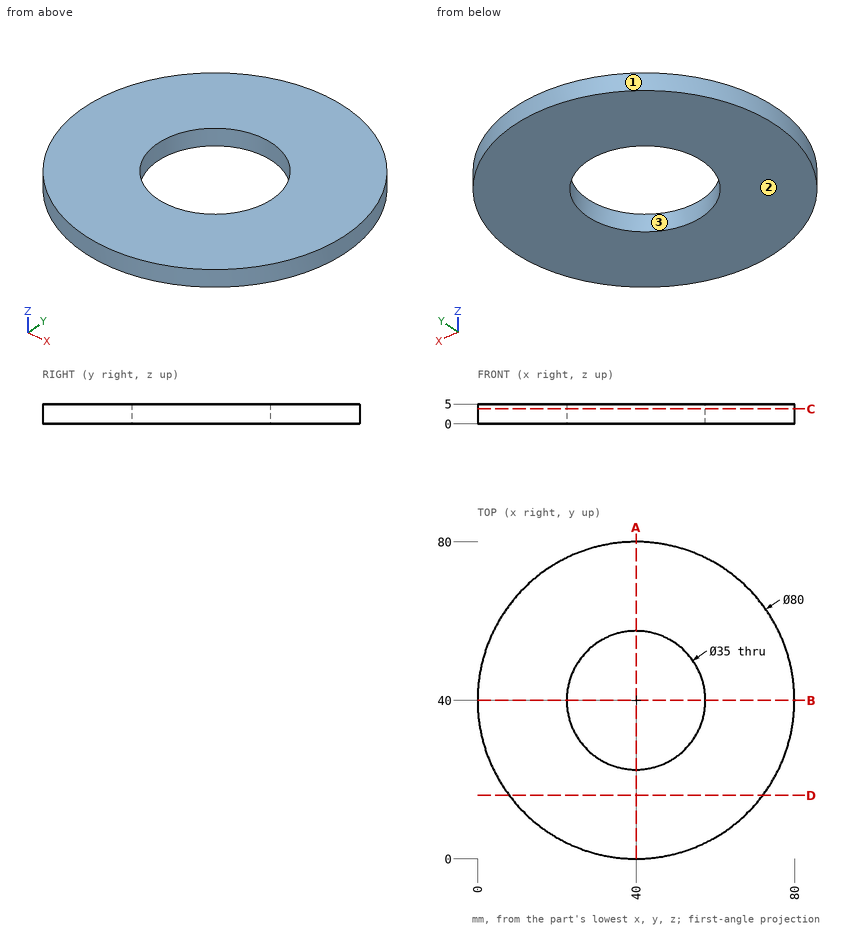
Print and shaded views of the part. All mm, measured from the part's lowest x, y and z. Round coordinates to 2 decimals unless told otherwise and drop trailing zeros. Write each loop counter-clockwise with the first axis right and the second up, starting at its lowest first coordinate (ties: lowest second). Pieces come first, ordered by that corner, then holes. Notation, with made-up numbers: (52.5, 32.25) - (81.5, 32.25) arc R22 ccw to (81.5, 52.25) - close; hole circle Ø7 at (7, -32). An arc over 180 degrees is marked (long way). Write each question's results on one line, items separated by ' | '. Start each with the question number.
Item 1: Drop flat-ended pins along their axis: P1, Ø1, axis at y = 17.5, z = 4, coming from the +X side; P2, Ø1.5, axis at y = 11.5, z = 1.5, coming from the -X side; P3, Ø1.5, axis at x = 34, z = 1, coming from the +Y side. Give the stop position or say it passes through.
Item 2: Saw through at A-A (x = 40). Write the cut outline in (y, z), and give its area (3 significant figures).
Item 3: Mould opens along Y. For the marked faces 1, 2 and 3 say: pulls with the +Y half, pulls with the -Y half, needs draft (parallel to the pull), parting line crosses it, or undercut.
Item 4: Saw through at C-C (z = 3.75). Write the cut outline in (x, y), and give its area (3 significant figures).
Item 5: Saw through at D-D (y = 16). Write the cut outline in (x, z).
Item 6: Wall check: L1, parallel to Y at x = 40, z = 1.25; L2, parallel to X at y = 50.5, z = 2.35; L3, parallel to X at y = 55.5, z = 3.5. Give the ranges that are in metal, low to high. Write a range as [from, to].
Results are:
1) P1: stops at x = 73.41 | P2: stops at x = 11.19 | P3: stops at y = 79.65
2) outline: (0, 0) - (22.5, 0) - (22.5, 5) - (0, 5) - close; (57.5, 0) - (80, 0) - (80, 5) - (57.5, 5) - close | area: 225 mm²
3) face 1: parting line crosses it | face 2: needs draft | face 3: undercut
4) outline: circle Ø80 at (40, 40); hole circle Ø35 at (40, 40) | area: 4,060 mm²
5) outline: (8, 0) - (72, 0) - (72, 5) - (8, 5) - close
6) L1: y = [0, 22.5], [57.5, 80] | L2: x = [1.4, 26], [54, 78.6] | L3: x = [3.13, 31.88], [48.12, 76.87]
